Read the model definition and answer for the solid it produces. Units are mm, in the model's axes. A direction names the side the tool comes from. Give positions to 0.01 mm unless a question says otherwise; leave off trailing zeros. Loops run counter-clockwise (first coordinate to the right, second up) from the corner with the lowest first, then second, coordinate; pieces in that order, holes last. Notation, with made-up numbers: (36.25, 61) - (59.25, 61) arc R20 ccw to (59.25, 66) - close; hole circle Ø10 at (-3.5, 49.5). An arc over 180 degrees is marked (long way). Write each question's results on one line, items separated by ' | '. Start each with the question number.
Q1. For faces 1 (the flat face through (1, 6, 89.5)), 2 (the flat face through (0, 5.464, 70)), determine the directions among +Z, -Z, +X, -X, +Y, -Y from which every point of the face is accessible in a straight line to the end or side of a thin tool.
Q2. The part is cut by section B-B, the plane y = -4. Write down the section's boundary in (x, z).
Q3. The part is cut by section D-D, the plane y = 17. Write down the section's boundary in (x, z).
Q4. Determine the mould class of faces 3 (the cylindrical face through (0.264, -2.141, 75.494)), 4 (the flat face through (15.773, -2, 1)), 5 (the flat face through (-14.227, -2, 1)), 6 (the cylindrical face through (0.264, -2.141, -63.506)) for opening direction X: +X half, -X half, draft (parallel to the pull), parting line (faces both ways), or undercut.
Q5. Given pin 1 (1.5 mm diameter, centred on y = 16.5, z = 65, fed in from +X); pin 2 (4 mm diameter, centred on x = 12.5, z = -26.5, fed in from +Y); pin 3 (3.5 mm diameter, centred on x = -1, z = -71, fed in from -Y), each flat-ended and moving along its own axis, determine where each tip first touches the part or whether it passes through.
Q6. The part is cut by section C-C, the plane x = 2.25. Write down the section's boundary in (y, z), plus the area to 3 significant figures.
Q7. The part is cut by section A-A, the plane z = 69.5. Write down the section's boundary in (x, y).
Q8. Find the intervals of material crossed by line 1 (X direction, y = -6, z = -69.5); line 2 (X direction, y = 18.5, z = 0); line 3 (Y direction, x = 10.25, z = -19), in increasing order. Write a range as from..to.
```python
from build123d import *

# Parameters (mm, degrees)
SALIENTE_EXTRUIR1_DEPTH = 89.5
CROQUIS3_R              = 6
CORTAR_EXTRUIR1_DEPTH   = 15


with BuildPart() as part:
    # Croquis2 → Saliente-Extruir1 (new, symmetric)
    with BuildSketch(Plane.XY):
        with BuildLine():
            Line((-14.226804124, -9.536082474), (15.773195876, -9.536082474))
            Line((15.773195876, -9.536082474), (15.773195876, 5.463917526))
            ThreePointArc((15.773195876, 5.463917526), (0.773195876, 20.463917526), (-14.226804124, 5.463917526))
            Line((-14.226804124, 5.463917526), (-14.226804124, -9.536082474))
        make_face()
    extrude(amount=SALIENTE_EXTRUIR1_DEPTH, both=True)

    # Croquis3 → Cortar-Extruir1 (cut)
    with BuildSketch(Plane.XZ.offset(9.536082474)):
        with Locations(Location((0, 69.5, 0), (0, 0, 270))):
            Circle(CROQUIS3_R)
        with Locations(Location((0, -69.5, 0), (0, 0, 270))):
            Circle(CROQUIS3_R)
    extrude(amount=-CORTAR_EXTRUIR1_DEPTH, mode=Mode.SUBTRACT)


solid = part.part
```
Check sheet entries:
1) face 1: +Z, +X, -X, +Y, -Y | face 2: -Y
2) outline: (-14.23, -89.5) - (15.77, -89.5) - (15.77, 89.5) - (-14.23, 89.5) - close; hole circle Ø12 at (0, -69.5); hole circle Ø12 at (0, 69.5)
3) outline: (-8.81, -89.5) - (10.36, -89.5) - (10.36, 89.5) - (-8.81, 89.5) - close
4) face 3: undercut | face 4: +X half | face 5: -X half | face 6: undercut
5) pin 1: stops at x = 11.69 | pin 2: stops at y = 16.88 | pin 3: stops at y = 5.46
6) outline: (-9.54, -89.5) - (20.39, -89.5) - (20.39, 89.5) - (-9.54, 89.5) - (-9.54, 75.06) - (5.46, 75.06) - (5.46, 63.94) - (-9.54, 63.94) - (-9.54, -63.94) - (5.46, -63.94) - (5.46, -75.06) - (-9.54, -75.06) - close | area: 5,020 mm^2
7) outline: (-14.23, -9.54) - (-6, -9.54) - (-6, 5.46) - (6, 5.46) - (6, -9.54) - (15.77, -9.54) - (15.77, 5.46) arc R15 ccw to (-14.23, 5.46) - close
8) line 1: x = -14.23..-6, 6..15.77 | line 2: x = -6.65..8.19 | line 3: y = -9.54..17.09
